Can you work these out from the drawing? Everything is in mm from the part's minimum corner. Give positions to 0.01 mm unless a question says otherwise; leave off trailing zeros. Write each loop counter-clockwise with the first axis right and the second up, starting at its lowest first coordinate (ties: lowest second). Pieces come first, ordered by that corner, then holes. Notation, with made-up numbers: (-11.75, 18) - (47.25, 18) arc R19 cw to (47.25, 44) - close; hole circle Ø9 at (36.5, 13). An arc over 180 degrees is marked (long way). Use a Markdown table: item, result.
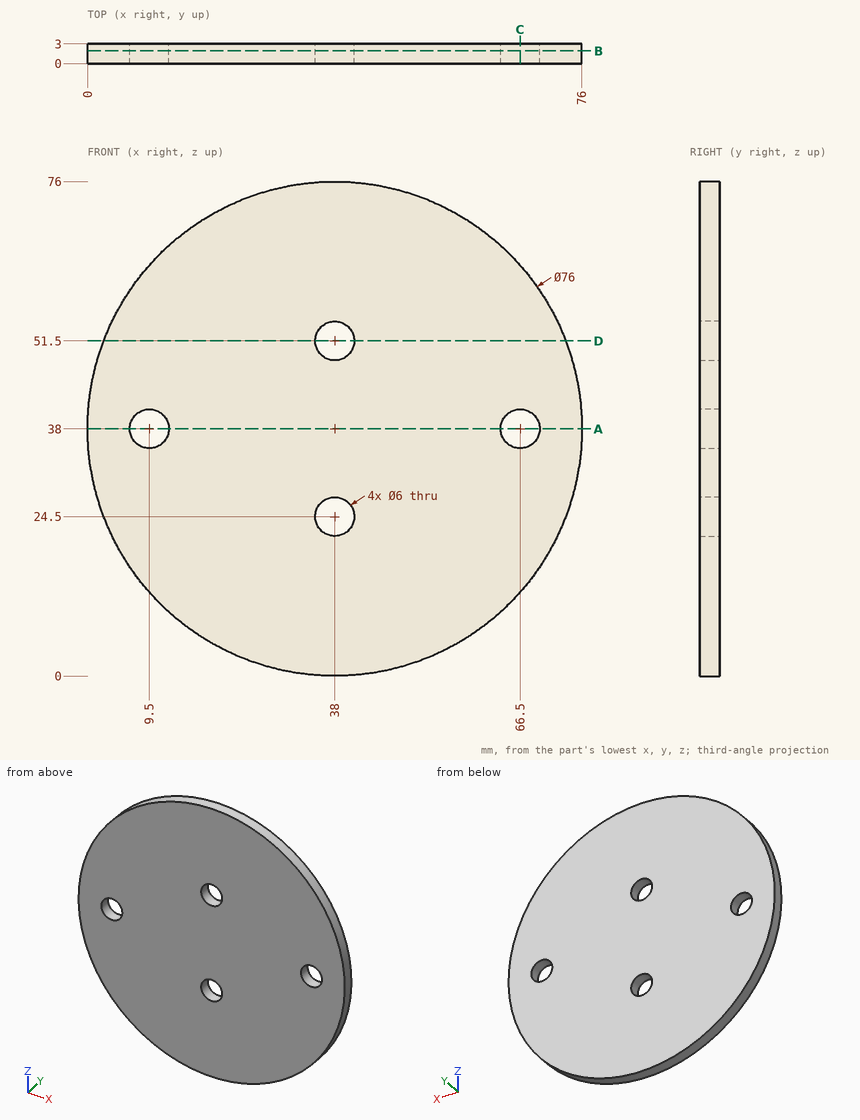
Item 1: I need wall thicknesses on line 1 along X through (y, z) = (1.2, 38); line 2 along X through (y, z) = (1.2, 51.5); line 3 along Z through (x, y) = (9, 1.7). Which ranges of each line are inside material? Lowest first, please. Write a range as [from, to].
Values:
| item | result |
|---|---|
| line 1 | x = [0, 6.5], [12.5, 63.5], [69.5, 76] |
| line 2 | x = [2.48, 35], [41, 73.52] |
| line 3 | z = [13.44, 35.04], [40.96, 62.56] |
Item 2: If we section it at D-D, the plane z = 51.5: Write out the boundary of the cut face in (x, y).
Values:
| item | result |
|---|---|
| outline | (2.48, 0) - (35, 0) - (35, 3) - (2.48, 3) - close; (41, 0) - (73.52, 0) - (73.52, 3) - (41, 3) - close |
Item 3: If we section it at C-C, the plane x = 66.5: Write out the boundary of the cut face in (y, z), plus the area to 3 significant figures.
Values:
| item | result |
|---|---|
| outline | (0, 12.87) - (3, 12.87) - (3, 35) - (0, 35) - close; (0, 41) - (3, 41) - (3, 63.13) - (0, 63.13) - close |
| area | 133 mm2 |
Item 4: If we section it at B-B, the plane y = 1.95: Write out the boundary of the cut face in (x, z), plus the area to 3 significant figures.
Values:
| item | result |
|---|---|
| outline | circle Ø76 at (38, 38); hole circle Ø6 at (9.5, 38); hole circle Ø6 at (38, 24.5); hole circle Ø6 at (38, 51.5); hole circle Ø6 at (66.5, 38) |
| area | 4,420 mm2 |
Item 5: If we section it at A-A, the plane z = 38: Write out the boundary of the cut face in (x, y), plus the area to 3 significant figures.
Values:
| item | result |
|---|---|
| outline | (0, 0) - (6.5, 0) - (6.5, 3) - (0, 3) - close; (12.5, 0) - (63.5, 0) - (63.5, 3) - (12.5, 3) - close; (69.5, 0) - (76, 0) - (76, 3) - (69.5, 3) - close |
| area | 192 mm2 |
